```python
from build123d import *

# Parameters (mm, degrees)
F1_DEPTH = 25.4
F3_DEPTH = 25.401
F5_DEPTH = 4.7625
F6_R     = 2.286
F7_DEPTH = 20.121


with BuildPart() as f1:
    # F0 (on Right) → F1 (new body)
    with BuildSketch(Plane.YZ):
        with BuildLine():
            ThreePointArc((1.27, 12.435317), (0, -12.5), (-1.27, 12.435317))
            Line((-1.27, 12.435317), (-1.27, 22.969053))
            Line((-1.27, 22.969053), (-4.445, 22.969053))
            Line((-4.445, 22.969053), (-4.445, 15.031553))
            ThreePointArc((-4.445, 15.031553), (-15.421435, 2.808021), (-9.458098, -12.5))
            Line((-9.458098, -12.5), (-25.4, -12.5))
            Line((-25.4, -12.5), (-25.4, -17.2625))
            Line((-25.4, -17.2625), (25.4, -17.2625))
            Line((25.4, -17.2625), (25.4, -12.5))
            Line((25.4, -12.5), (9.458098, -12.5))
            ThreePointArc((9.458098, -12.5), (15.421435, 2.808021), (4.445, 15.031553))
            Line((4.445, 15.031553), (4.445, 22.969053))
            Line((4.445, 22.969053), (1.27, 22.969053))
            Line((1.27, 22.969053), (1.27, 12.435317))
        make_face()
    extrude(amount=F1_DEPTH)

    # F2 (on face) → F3 (cut, through all)
    with BuildSketch(Plane(origin=(0, 0, 0), x_dir=(0, -1, 0), z_dir=(-1, 0, 0))):
        Polygon((25.4, -12.5), (9.458098, -12.5), (3.163889, -17.2625), (25.4, -17.2625), align=None)
    extrude(amount=-F3_DEPTH, mode=Mode.SUBTRACT)

    # F4 (on face) → F5 (cut, through all)
    with BuildSketch(Plane.XY.offset(-12.5)):
        with BuildLine():
            Line((4.6609, 25.4), (4.6609, 17.4625))
            ThreePointArc((4.6609, 17.4625), (6.35, 15.7734), (8.0391, 17.4625))
            Line((8.0391, 17.4625), (8.0391, 25.4))
            Line((8.0391, 25.4), (4.6609, 25.4))
        make_face()
        with BuildLine():
            Line((17.3609, 25.4), (17.3609, 17.4625))
            ThreePointArc((17.3609, 17.4625), (19.05, 15.7734), (20.7391, 17.4625))
            Line((20.7391, 17.4625), (20.7391, 25.4))
            Line((20.7391, 25.4), (17.3609, 25.4))
        make_face()
    extrude(amount=-F5_DEPTH, mode=Mode.SUBTRACT)

    # F6 (on face) → F7 (cut, through all)
    with BuildSketch(Plane(origin=(0, 4.445, 0), x_dir=(-1, 0, 0), z_dir=(0, 1, 0))):
        with Locations((-19.05, 19.000303)):
            Circle(F6_R)
        with Locations((-6.35, 19.000303)):
            Circle(F6_R)
    extrude(amount=-F7_DEPTH, mode=Mode.SUBTRACT)


solid = f1.part
```
Geometry: final body of the model. Coordinates: model frame, mm. A direction names the side the tool comes from. Coordinates: 2 decimals unless noted, no trailing zeros. Order: outer loops, then holes, each group sorted by start corner. A loop starts at its lowest first (then second) coordinate and runs counter-clockwise, first axis right, second up. Notation, with made-up numbers: (-16, 76) - (23, 76) arc R30 cw to (23, 108) - close; hole circle Ø10 at (16, 78.5). An arc over 180 degrees is marked (long way). Return JSON: item names as keys, results as strings. Group by question number.
1. Pin query (flat end, axial travel): pin 1 (13 mm diameter, centred on x = 17, y = 16, fed in from +Z); pin 2 (3 mm diameter, centred on x = 10.5, z = 15, fed in from -Y); pin 3 (5.5 mm diameter, centred on x = 19.05, z = 19, fed in from +Y) (3 decimals). Return the tip coordinate at first contact, or that it passes through.
2. Cut plane B-B (x = 19.05). Count the separate pieces of the cut face and the enclosed holes in it, plus the area to 3 significant figures.
3. Cut plane C-C (y = 20.5). Output: boundary loops of the cut face in (x, z), plus the area to 3 significant figures.
4. Cut plane D-D (y = -7.5). Output: boundary loops of the cut face in (x, z), plus the area to 3 significant figures.
5. Set-up query: faces 1 (the face through (13, -4.445, 19)), 2 (the face through (0, 12.4, -3)), 3 (the face through (13, 4.445, 19)), 4 (the face through (4.661, 21, -15)), 5 (the face through (13, 25.4, -15)). Return all of +Z, -Z, +X, -X, +Y, -Y with unobstructed straight access to the full face (end or side cutting, diameter ignored); none if empty.
6. Material intervals for line 1 along Z through (x, y) = (19.05, -3.2); line 2 along Z through (x, y) = (17.25, 11); line 3 along Y through (x, z) = (11.5, 8), sorted ascending. Write a range as [from, to].
7. Pull-direction query (Y, two-part tool) for faces 6 (the face through (13, 1.27, 18)), 7 (the face through (2, 25.4, -15)), 8 (the face through (17.361, 21, -15)); classes: pulls with the +Y half, pulls with the -Y half, needs draft (parallel to the pull), parting line crosses it, or undercut.
8. Cut plane A-A (z = 0). Output: boundary loops of the cut face in (x, y) (3 decimals), plus the area to 3 significant figures.
Resolved:
{
 "1": {"pin 1": "stops at z = 12.47", "pin 2": "stops at y = -7.97", "pin 3": "stops at y = 4.445"},
 "2": {"separate pieces": "3", "enclosed holes": "0", "area": "356 mm²"},
 "3": {"outline": "(0, -17.26) - (4.66, -17.26) - (4.66, -12.5) - (0, -12.5) - close; (8.04, -17.26) - (17.36, -17.26) - (17.36, -12.5) - (8.04, -12.5) - close; (20.74, -17.26) - (25.4, -17.26) - (25.4, -12.5) - (20.74, -12.5) - close", "area": "88.8 mm²"},
 "4": {"outline": "(0, -13.98) - (25.4, -13.98) - (25.4, -10) - (0, -10) - close; (0, 10) - (25.4, 10) - (25.4, 13.76) - (0, 13.76) - close", "area": "197 mm²"},
 "5": {"face 1": "+Z, +X, -X, -Y", "face 2": "+Z, -Z, -X, +Y, -Y", "face 3": "+Z, +X, -X, +Y", "face 4": "+Z, -Z, +Y", "face 5": "+Z, -Z, +X, -X, +Y"},
 "6": {"line 1": "z = [-17.24, -12.08], [12.08, 16.71], [21.29, 22.97]", "line 2": "z = [-17.26, -12.5], [-11.17, -5.94], [5.94, 11.17]", "line 3": "y = [-13.48, -9.6], [9.6, 13.48]"},
 "7": {"face 6": "undercut", "face 7": "pulls with the +Y half", "face 8": "needs draft"},
 "8": {"outline": "(0, -15.675) - (25.4, -15.675) - (25.4, -12.5) - (0, -12.5) - close; (0, 12.5) - (25.4, 12.5) - (25.4, 15.675) - (0, 15.675) - close", "area": "161 mm²"}
}
